CAD build for the part. Positions are in the model's coordinates, mm. Face numbers are marked on the shaded views. Round coordinates to 2 decimals unless told otherwise and drop trailing zeros. Order: outer loops, then holes, each group sorted by start corner. A loop starts at its lowest first (then second) coordinate and runs counter-clockwise, first axis right, second up. Notation, with made-up numbers: M 81.25,78.5 L 127.25,78.5 A4 ccw 127.25,84.5 Z; hole C 66.5,-15 d5. An arc over 180 degrees is marked long. Answer as a JSON object with one key per item and string values.
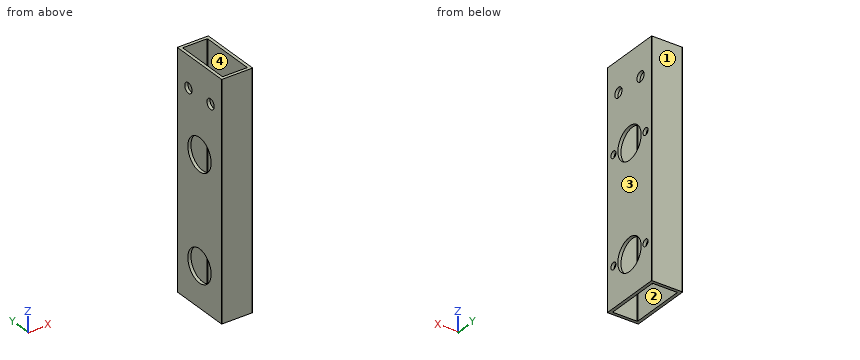
```python
from build123d import *

# Parameters (mm, degrees)
EXTRUDE_1_DEPTH     = 150
SKETCH_2_R          = 3.25
CUT_EXTRUDE_1_DEPTH = 157.524758425
SKETCH_3_R          = 10.5
CUT_EXTRUDE_2_DEPTH = 157.524758425
SKETCH_4_R          = 10.5
CUT_EXTRUDE_3_DEPTH = 157.524758425
SKETCH_5_R          = 2.25
CUT_EXTRUDE_4_DEPTH = 10
SKETCH_5_4_R        = 2.25
CUT_EXTRUDE_5_DEPTH = 10


with BuildPart() as part:
    # ｽｹｯﾁ1 → ﾎﾞｽ - 押し出し1 (new body)
    with BuildSketch(Plane.XY):
        with BuildLine():
            Line((0.3, 0), (19.7, 0))
            ThreePointArc((19.7, 0), (19.912132034, 0.087867966), (20, 0.3))
            Line((20, 0.3), (20, 39.7))
            ThreePointArc((20, 39.7), (19.912132034, 39.912132034), (19.7, 40))
            Line((19.7, 40), (0.3, 40))
            ThreePointArc((0.3, 40), (0.087867966, 39.912132034), (0, 39.7))
            Line((0, 39.7), (0, 0.3))
            ThreePointArc((0, 0.3), (0.087867966, 0.087867966), (0.3, 0))
        make_face()
        with BuildLine():
            Line((2.3, 2), (17.7, 2))
            ThreePointArc((17.7, 2), (17.912132034, 2.087867966), (18, 2.3))
            Line((18, 2.3), (18, 37.7))
            ThreePointArc((18, 37.7), (17.912132034, 37.912132034), (17.7, 38))
            Line((17.7, 38), (2.3, 38))
            ThreePointArc((2.3, 38), (2.087867966, 37.912132034), (2, 37.7))
            Line((2, 37.7), (2, 2.3))
            ThreePointArc((2, 2.3), (2.087867966, 2.087867966), (2.3, 2))
        make_face(mode=Mode.SUBTRACT)
    extrude(amount=-EXTRUDE_1_DEPTH)

    # ｽｹｯﾁ2 → ｶｯﾄ - 押し出し1 (cut, through all)
    with BuildSketch(Plane.ZY):
        with Locations((-20, 30)):
            Circle(SKETCH_2_R)
        with Locations((-20, 10)):
            Circle(SKETCH_2_R)
    extrude(amount=-CUT_EXTRUDE_1_DEPTH, mode=Mode.SUBTRACT)

    # ｽｹｯﾁ3 → ｶｯﾄ - 押し出し2 (cut, through all)
    with BuildSketch(Plane(origin=(20, 0, 0), x_dir=(0, 0, -1), z_dir=(1, 0, 0))):
        with Locations((124.125, 20)):
            Circle(SKETCH_3_R)
    extrude(amount=-CUT_EXTRUDE_2_DEPTH, mode=Mode.SUBTRACT)

    # ｽｹｯﾁ4 → ｶｯﾄ - 押し出し3 (cut, through all)
    with BuildSketch(Plane(origin=(20, 0, 0), x_dir=(0, 0, -1), z_dir=(1, 0, 0))):
        with Locations((55.875, 20)):
            Circle(SKETCH_4_R)
    extrude(amount=-CUT_EXTRUDE_3_DEPTH, mode=Mode.SUBTRACT)

    # ｽｹｯﾁ5 → ｶｯﾄ - 押し出し4 (cut)
    with BuildSketch(Plane(origin=(20, 0, 0), x_dir=(0, 0, -1), z_dir=(1, 0, 0))):
        with Locations((124.125, 5.5)):
            Circle(SKETCH_5_R)
    extrude(amount=-CUT_EXTRUDE_4_DEPTH, mode=Mode.SUBTRACT)

    # ｽｹｯﾁ5<4> → ｶｯﾄ - 押し出し5 (cut)
    with BuildSketch(Plane(origin=(20, 0, 0), x_dir=(0, 0, -1), z_dir=(1, 0, 0))):
        with Locations((55.875, 34.5)):
            Circle(SKETCH_5_4_R)
        with Locations((55.875, 5.5)):
            Circle(SKETCH_5_4_R)
        with Locations((124.125, 5.5)):
            Circle(SKETCH_5_4_R)
        with Locations((124.125, 34.5)):
            Circle(SKETCH_5_4_R)
    extrude(amount=-CUT_EXTRUDE_5_DEPTH, mode=Mode.SUBTRACT)


solid = part.part
```
Item 1: Wall check: line 1 along Y through (x, z) = (12, -122.5); line 2 along X through (y, z) = (30, -89). Give the ranges that are in metal, low to high. Write a range as [from, to].
Worked answers:
{"line 1": "y = [0, 2], [38, 40]", "line 2": "x = [0, 2], [18, 20]"}
Item 2: Two-plate mould, pull along X, no slides. Class the marked faces 1, 2, 3 and 4: released by +X, released by -X, zero draft, split by the parting line, or undercut.
Worked answers:
{"face 1": "zero draft", "face 2": "undercut", "face 3": "released by +X", "face 4": "undercut"}
Item 3: Saw through at D-D on z = -120. List the corners of the cut face in (x, y), and give its area (3 significant figures).
Worked answers:
{"outline": "M 0,0.3 A0.3 ccw 0.3,0 L 19.7,0 A0.3 ccw 20,0.3 L 20,10.34 L 18,10.34 L 18,2.3 A0.3 cw 17.7,2 L 2.3,2 A0.3 cw 2,2.3 L 2,10.34 L 0,10.34 Z; M 0,29.66 L 2,29.66 L 2,37.7 A0.3 cw 2.3,38 L 17.7,38 A0.3 cw 18,37.7 L 18,29.66 L 20,29.66 L 20,39.7 A0.3 ccw 19.7,40 L 0.3,40 A0.3 ccw 0,39.7 Z", "area": "147 mm2"}
Item 4: Saw through at B-B on z = -20. State how many separate pieces and enclosed holes the cut face has, and give its area (3 significant figures).
Worked answers:
{"separate pieces": "4", "enclosed holes": "0", "area": "172 mm2"}
Item 5: Saw through at A-A on x = 5.5. List the corners of the cut face in (y, z), and give its area (3 significant figures).
Worked answers:
{"outline": "M 0,-150 L 2,-150 L 2,0 L 0,0 Z; M 38,-150 L 40,-150 L 40,0 L 38,0 Z", "area": "600 mm2"}
Item 6: Drop flat-ended pins along their axis: pin 1 Ø3.5 at (y, z) = (5.5, -55.875) entering from +X; pin 2 Ø4 at (y, z) = (10, -20) entering from -X. Give the stop position or say it passes through.
Worked answers:
{"pin 1": "stops at x = 2", "pin 2": "passes through"}
Item 7: Saw through at C-C on y = 20. List the corners of the cut face in (x, z) (3 decimals).
Worked answers:
{"outline": "M 0,-150 L 2,-150 L 2,-134.625 L 0,-134.625 Z; M 0,-113.625 L 2,-113.625 L 2,-66.375 L 0,-66.375 Z; M 0,-45.375 L 2,-45.375 L 2,0 L 0,0 Z; M 18,-150 L 20,-150 L 20,-134.625 L 18,-134.625 Z; M 18,-113.625 L 20,-113.625 L 20,-66.375 L 18,-66.375 Z; M 18,-45.375 L 20,-45.375 L 20,0 L 18,0 Z"}
